from build123d import *

# Parameters (mm, degrees)
SKETCH_1_R          = 2.9
EXTRUDE_1_DEPTH     = 4
SKETCH_2_W          = 12.628096459
SKETCH_2_H          = 3.5
EXTRUDE_2_DEPTH     = 1
SKETCH_3_R          = 0.5
SKETCH_3_R_2        = 1
CUT_EXTRUDE_1_DEPTH = 5
FILLET_1_R          = 1.5
SKETCH_4_R          = 1.9
CUT_EXTRUDE_2_DEPTH = 3


with BuildPart() as part:
    # 草图1 → 凸台-拉伸1 (new body)
    with BuildSketch(Plane(origin=(0, 0, 0), x_dir=(1, 0, 0), z_dir=(0, 1, 0))):
        Circle(SKETCH_1_R)
    extrude(amount=EXTRUDE_1_DEPTH)

    # 草图2 → 凸台-拉伸2 (add)
    with BuildSketch(Plane(origin=(0, 0, 0), x_dir=(1, 0, 0), z_dir=(0, 1, 0))):
        with Locations((7.685951771, 0)):
            Rectangle(SKETCH_2_W, SKETCH_2_H)
    extrude(amount=EXTRUDE_2_DEPTH)

    # 草图3 → 切除-拉伸1 (cut, through all)
    with BuildSketch(Plane(origin=(0, 0, 0), x_dir=(1, 0, 0), z_dir=(0, 1, 0))):
        with Locations((8, 0)):
            Circle(SKETCH_3_R)
        with Locations((12, 0)):
            Circle(SKETCH_3_R)
        with Locations((10, 0)):
            Circle(SKETCH_3_R)
        Circle(SKETCH_3_R_2)
    extrude(amount=CUT_EXTRUDE_1_DEPTH, mode=Mode.SUBTRACT)

    # 圆角1
    fillet_1_edges = [part.edges().sort_by_distance(p)[0] for p in [
        (14, 0.5, -1.75),
        (14, 0.5, 1.75),
    ]]
    fillet(fillet_1_edges, radius=FILLET_1_R)

    # 草图4 → 切除-拉伸2 (cut)
    with BuildSketch(Plane(origin=(0, 4, 0), x_dir=(1, 0, 0), z_dir=(0, 1, 0))):
        Circle(SKETCH_4_R)
    extrude(amount=-CUT_EXTRUDE_2_DEPTH, mode=Mode.SUBTRACT)


solid = part.part
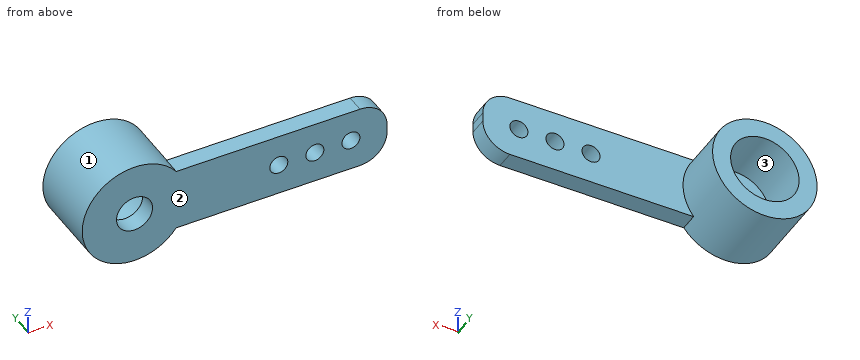
Geometry check sheet. Reference: the model listing, model coordinates, mm. Face numbers are marked on the shaded views. Give positions to 0.01 mm unless a question says otherwise; leave off trailing zeros. Write each loop counter-clockwise with the first axis right and the second up, starting at its lowest first coordinate (ties: lowest second). Pieces come first, ordered by that corner, then holes. Notation, with made-up numbers: M -17,58.25 L 35,58.25 A35 cw 35,91.25 Z; hole C 75.5,-6 d4. An arc over 180 degrees is marked long. Answer as CSV lines item,"result". Start each with the question number.
Q1. Go/stop test with flat-tipped pins: pin 1 (1.8 mm diameter, centred on x = 0, z = 0, fed in from -Y); pin 2 (2 mm diameter, centred on y = 2.5, z = 2, fed in from -X); pin 3 (1.8 mm diameter, centred on x = 8.5, z = -0.5, fed in from +Y); pin 4 (0.5 mm diameter, centred on x = 9.5, y = 0.5, fed in from -Z). Record where each tip stops, or that it passes through.
Q2. Material ranges on L1, parallel to X at y = 0.75, z = 0; L2, parallel to Z at x = 0, y = 2.6; L3, parallel to Z at x = 10, y = 0.2, recorded low to high.
Q3. Section check B-B, the plane y = 0.3. Record the cut outline in (x, z).
Q4. Section check A-A, the plane x = 8. Record the cut outline in (y, z), then the cut area to 3 significant figures.
Q5. Section check C-C, the plane z = 0. Record the cut outline in (x, y).
Q6. Section check D-D, the plane y = 2.1. Record the cut outline in (x, z).
Q7. Release check for a two-part mould opening along X. For the marked faces 1, 2 and 3 record: pulls with the +X half, pulls with the -X half, needs draft (parallel to the pull), parting line crosses it, or undercut.
Geometry says:
1,pin 1,"through"
1,pin 2,"x = -2.72"
1,pin 3,"y = 1"
1,pin 4,"z = -1.75"
2,L1,"-2.9 to -1, 1 to 7.5, 8.5 to 9.5, 10.5 to 11.5, 12.5 to 14"
2,L2,"-2.9 to -1.9, 1.9 to 2.9"
2,L3,"-1.75 to -0.5, 0.5 to 1.75"
3,outline,"M 2.31,-1.75 L 12.5,-1.75 A1.5 ccw 14,-0.25 L 14,0.25 A1.5 ccw 12.5,1.75 L 2.31,1.75 A2.9 ccw long Z; hole C 0,0 d2; hole C 8,0 d1; hole C 10,0 d1; hole C 12,0 d1"
4,outline,"M 0,-1.75 L 1,-1.75 L 1,-0.5 L 0,-0.5 Z; M 0,0.5 L 1,0.5 L 1,1.75 L 0,1.75 Z"
4,area,"2.50 mm^2"
5,outline,"M -2.9,0 L -1,0 L -1,1 L -1.9,1 L -1.9,4 L -2.9,4 Z; M 1,0 L 7.5,0 L 7.5,1 L 2.9,1 L 2.9,4 L 1.9,4 L 1.9,1 L 1,1 Z; M 8.5,0 L 9.5,0 L 9.5,1 L 8.5,1 Z; M 10.5,0 L 11.5,0 L 11.5,1 L 10.5,1 Z; M 12.5,0 L 14,0 L 14,1 L 12.5,1 Z"
6,outline,"C 0,0 d5.8; hole C 0,0 d3.8"
7,face 1,"parting line crosses it"
7,face 2,"needs draft"
7,face 3,"undercut"
